Autodesk Inventor part; units mm, degrees
ref_plane "YZ Plane" through (0, 0, 0) normal (1, 0, 0) x (0, 1, 0)
ref_plane "XZ Plane" through (0, 0, 0) normal (0, 1, 0) x (-1, 0, 0)
ref_plane "XY Plane" through (0, 0, 0) normal (0, 0, 1) x (1, 0, 0)
sketch "Sketch1" plane through (0, 0, 0) normal (1, 0, 0) x (0, 1, 0)
  line L0 (10.7218, 19.6361) -> (-10.1869, 19.6361)
  line L1 (-10.1869, 19.6361) -> (-10.1869, -15.2669)
  line L2 (10.7218, -15.2889) -> (10.7218, 19.6361)
  line L3 (10.7218, -15.2889) -> (15.8018, -15.2889)
  line L4 (15.8018, -15.2889) -> (15.8018, -19.2513)
  line L5 (15.8018, -19.2513) -> (-10.1869, -19.2513)
  line L6 (-10.1869, -15.2669) -> (-10.1869, -19.2513)
  line L7 (15.8018, -19.2513) -> (-11.1857, -19.2513) construction
  line L8 (-10.1869, -19.2513) -> (-10.1869, 35.0894) construction
  point P0 (0, 0)
  dimension "d0" = 3.9624
  dimension "d1" = 38.8874
  dimension "d2" = 5.08
  dimension "d4" = 26.9875
revolve "Revolution1" add sketch "Sketch1" angle 360 about axis through (0, -10.1869, -19.2513) along (0, 0, 1)
sketch "Sketch2" plane through (0, -10.1869, 19.6361) normal (0, 0, 1) x (1, 0, 0)
  point P0 (0, 10.1869)
  point P1 (0, 0)
hole "Hole1" at (0, -10.1869, 19.6361) direction (0, 0, -1) diameter 4.9784 depth 25.4 tip angle 118
fillet "Fillet1" radius 0.7874 1 edges at (0, -36.1756, -19.2513)
properties part number "lower die 1 center" material "Steel"
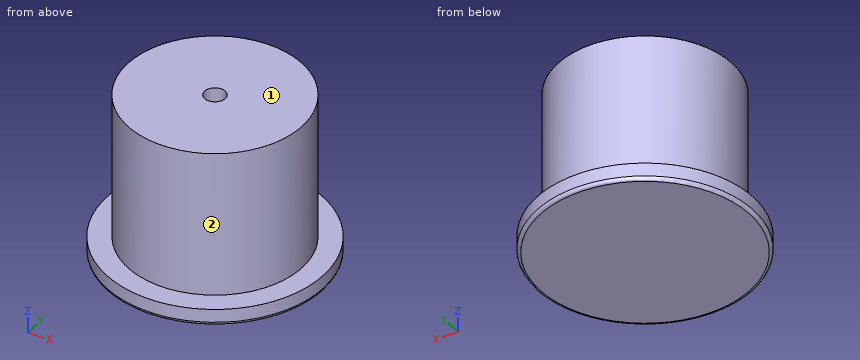
Can you work these out from the model? Positions are in its coordinate system, mm. Face numbers are marked on the shaded views. A direction names the side the tool comes from. Round coordinates to 2 decimals unless told otherwise and drop trailing zeros. Loops run counter-clockwise (first coordinate to the right, second up) from the corner with the lowest first, then second, coordinate; pieces in that order, holes last. Notation, with made-up numbers: (74.25, -26) - (100.25, -26) arc R6 ccw to (100.25, -21) - close; hole circle Ø6 at (13.5, -6). An arc over 180 degrees is marked (long way). Answer in a Markdown table with one row per item. Add a question column.
Q1. Which directions (+Z, -Z, +X, -X, +Y, -Y) give clear straight access to the entire face, cutting with the end or side of a thin tool? Please do the marked faces 1 and 2.
Q2. I want a section at A-A on z = -3. List the corners of the cut face in (x, y) for me, and give its area (3 significant figures).
Q3. For pin 1 Ø10 at (y, z) = (-24.5, 12.5) entering from -X; pin 2 Ø2 at (y, z) = (3.5, -13.5) entering from +X; pin 3 Ø5 at (y, z) = (-15.5, 4.5) entering from +X; pin 4 Ø8 at (x, y) = (0, -10.19) entering from +Z, each with a flat end and sliding along its axis, tell me the tip position at first contact or that it passes through.
Q4. I need wall thicknesses on L1, parallel to Y at x = 0, z = 14; L2, parallel to X at y = -11, z = 5; L3, parallel to X at y = 5.5, z = 7.5. Which ranges of each line are inside material? Lowest first, please.
Q5. I want a section at B-B on z = -11.5. List the corners of the cut face in (x, y) for me.
A:
| question | item | result |
|---|---|---|
| 1 | face 1 | +Z, +X, -X, +Y, -Y |
| 1 | face 2 | +Z |
| 2 | outline | circle Ø41.82 at (0, -10.19); hole circle Ø4.98 at (0, -10.19) |
| 2 | area | 1,350 mm^2 |
| 3 | pin 1 | x = -18.72 |
| 3 | pin 2 | x = 16.62 |
| 3 | pin 3 | x = 20.72 |
| 3 | pin 4 | z = 19.64 |
| 4 | L1 | -31.1 to -12.68, -7.7 to 10.72 |
| 4 | L2 | -20.89 to -2.35, 2.35 to 20.89 |
| 4 | L3 | -13.82 to 13.82 |
| 5 | outline | circle Ø41.82 at (0, -10.19) |
